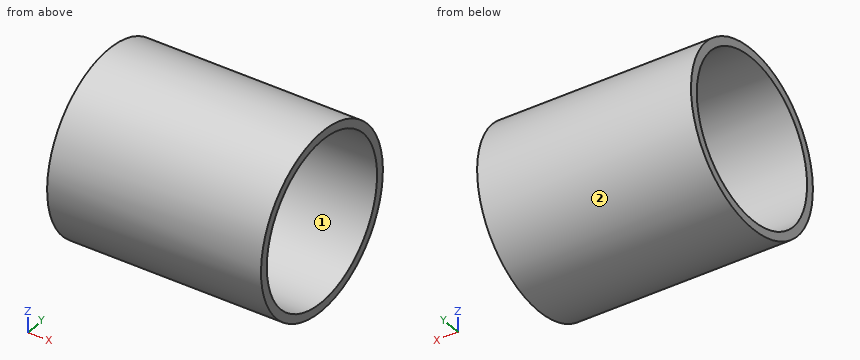
from build123d import *

# Parameters (mm, degrees)
CYLINDER009_R           = 9.5
CYLINDER009_DEPTH       = 25
CYLINDER009_PITCH_ANGLE = 90
CYLINDER007_R           = 10.5
CYLINDER007_DEPTH       = 25
CYLINDER007_PITCH_ANGLE = 90


with BuildPart() as cylinder007:
    # Cylinder009 → Cylinder009 (new body)
    with BuildSketch(Plane.XY):
        Circle(CYLINDER009_R)
    extrude(amount=CYLINDER009_DEPTH)


with BuildPart() as cylinder007_1:
    # Cylinder009 pitch: moved
    add(cylinder007.part.rotate(Axis((0, 0, 0), (0, 1, 0)), CYLINDER009_PITCH_ANGLE))


with BuildPart() as cylinder007_2:
    # Cylinder009 placement: moved
    add(cylinder007_1.part.moved(Location((156, 0, 0))))


with BuildPart() as cut004:
    # Cylinder007 → Cylinder007 (new body)
    with BuildSketch(Plane.XY):
        Circle(CYLINDER007_R)
    extrude(amount=CYLINDER007_DEPTH)


with BuildPart() as cut004_1:
    # Cylinder007 pitch: moved
    add(cut004.part.rotate(Axis((0, 0, 0), (0, 1, 0)), CYLINDER007_PITCH_ANGLE))


with BuildPart() as cut004_2:
    # Cylinder007 placement: moved
    add(cut004_1.part.moved(Location((156, 0, 0))))

    # Cut004: cut Cylinder007
    add(cylinder007_2.part, mode=Mode.SUBTRACT)


solid = cut004_2.part
The listing builds one solid part. Answer for the finished solid, in the listing's coordinates (mm). Face numbers are marked on the shaded views. Coordinates: 2 decimals unless noted, no trailing zeros. Loops run counter-clockwise (first coordinate to the right, second up) from the corner with the lowest first, then second, coordinate; pieces in that order, holes last.
1) Find the intervals of material crossed by L1, parallel to Y at x = 165, z = 0; L2, parallel to Z at x = 158.75, y = 6.75; L3, parallel to Y at x = 167.75, z = 5.75, in increasing order.
2) Find section A-A on z = 0. Write down the section's boundary in (x, y), then the cut area to 3 significant figures.
3) Determine the mould class of the marked faces 1 and 2 for opening direction Y: pulls with the +Y half, pulls with the -Y half, needs draft (parallel to the pull), parting line crosses it, or undercut.
4) Find section C-C on x = 173.75. Write down the section's boundary in (y, z), then the cut area to 3 significant figures.
5) Flat-ended cylindrical pins translate along their axes: pin 1 Ø6 at (x, z) = (166, 4.5) entering from +Y; pin 2 Ø8 at (x, y) = (162.5, 5) entering from -Z; pin 3 Ø6 at (x, y) = (165, -6) entering from -Z; pin 4 Ø2 at (x, z) = (176.5, 0.5) entering from +Y. Find the tip coordinate at first contact, or state that the pin passes through.
Values:
1. L1: y = -10.5 to -9.5, 9.5 to 10.5
1. L2: z = -8.04 to -6.68, 6.68 to 8.04
1. L3: y = -8.79 to -7.56, 7.56 to 8.79
2. outline: (156, -10.5) - (181, -10.5) - (181, -9.5) - (156, -9.5) - close; (156, 9.5) - (181, 9.5) - (181, 10.5) - (156, 10.5) - close
2. area: 50.0 mm2
3. face 1: undercut
3. face 2: parting line crosses it
4. outline: circle Ø21 at (0, 0); hole circle Ø19 at (0, 0)
4. area: 62.8 mm2
5. pin 1: stops at y = 10.39
5. pin 2: stops at z = -10.45
5. pin 3: stops at z = -10.06
5. pin 4: stops at y = 10.5
